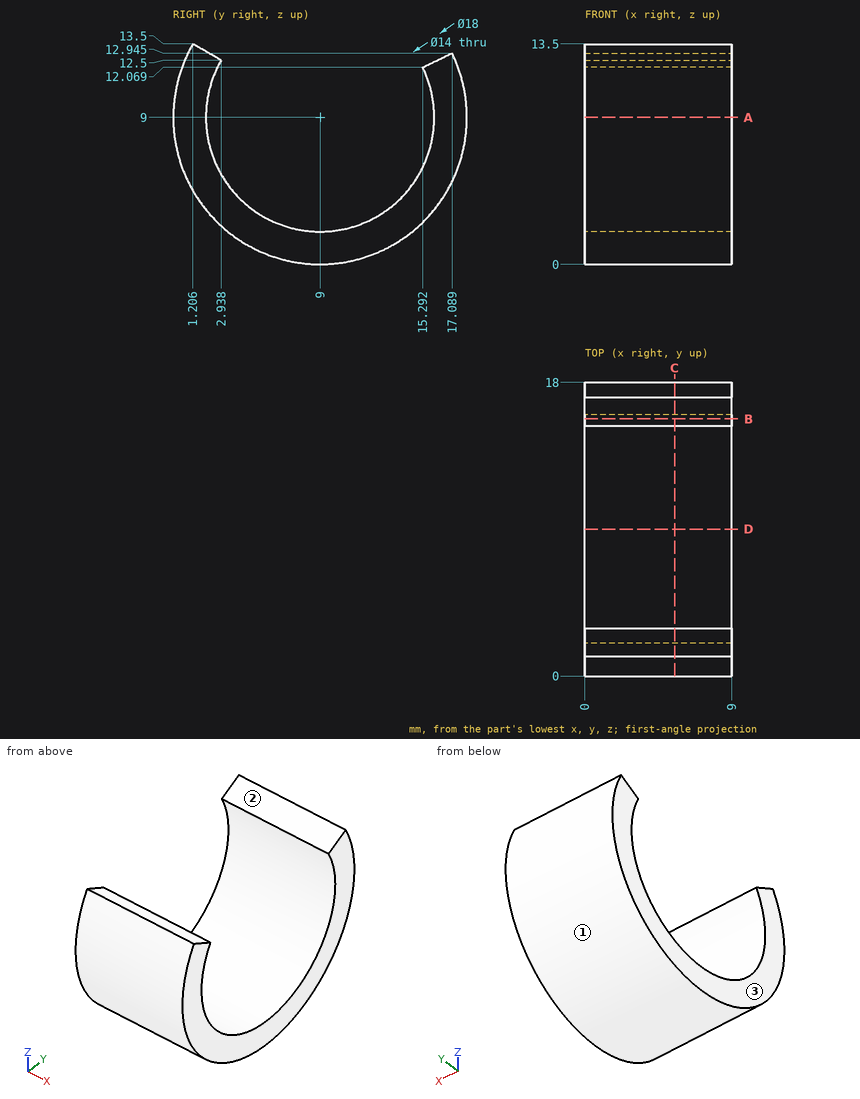
Here's the drawing with two shaded views (mm, measured from the low corner). I have some questions. Coordinates: 2 decimals unless noted, no trailing zeros. Order: outer loops, then holes, each group sorted by start corner. A loop starts at its lowest first (then second) coordinate and runs counter-clockwise, first axis right, second up. Notation, with made-up numbers: (-29, 70.5) - (17, 70.5) arc R23 cw to (17, 106.5) - close; hole circle Ø10 at (-26, -27.75). An arc over 180 degrees is marked (long way). Use CSV: the item, a comma, the result in double quotes. Start each with the question number.
1. Please list where these lines run through material, in increasing order: line 1 (Y direction, x = 4, z = 9); line 2 (Y direction, x = 4, z = 12.75) (1 decimal); line 3 (Z direction, x = 1.5, y = 9.25) (1 decimal). Write a range as from..to.
2. Suppose I cut it at A-A on z = 9. List the corners of the cut face in (x, y) for me, then the cut area to 3 significant figures.
3. Suppose I cut it at D-D on y = 9. List the corners of the cut face in (x, z) for me.
4. Suppose I cut it at B-B on y = 15.75. List the corners of the cut face in (x, z) for me.
5. I'm going to push flat-ended pins straight in: pin 1 (1 mm diameter, centred on x = 2, y = 2.5, fed in from -Z); pin 2 (2 mm diameter, centred on x = 3, y = 13.5, fed in from -Z); pin 3 (3 mm diameter, centred on x = 7, z = 1.5, fed in from +Y). Where does each tip first touch, or does it pass through?
6. Suppose I cut it at C-C on x = 5.5. List the corners of the cut face in (y, z) for me (1 decimal).
7. If we mould it in two halves opening along Y, with no side actions, what happens to the marked faces 1, 2 and 3? For each: +Y half, -Y half, draft (parallel to the pull), parting line (faces both ways), or undercut.
Output:
1,line 1,"y = 0..2, 16..18"
1,line 2,"y = 0.8..2.5, 16.7..17.2"
1,line 3,"z = 0..2"
2,outline,"(0, 0) - (9, 0) - (9, 2) - (0, 2) - close; (0, 16) - (9, 16) - (9, 18) - (0, 18) - close"
2,area,"36.0 mm2"
3,outline,"(0, 0) - (9, 0) - (9, 2) - (0, 2) - close"
4,outline,"(0, 3.05) - (9, 3.05) - (9, 7.15) - (0, 7.15) - close; (0, 10.85) - (9, 10.85) - (9, 12.29) - (0, 12.29) - close"
5,pin 1,"stops at z = 2.29"
5,pin 2,"stops at z = 0.71"
5,pin 3,"stops at y = 15.71"
6,outline,"(1.2, 13.5) arc R9 ccw (long way) to (17.1, 12.9) - (15.3, 12.1) arc R7 cw (long way) to (2.9, 12.5) - close"
7,face 1,"parting line"
7,face 2,"undercut"
7,face 3,"draft"
